Build history of the part. All positions in model axes, mm. A direction names the side the tool comes from. Give positions to 0.01 mm unless a question says otherwise; leave off trailing zeros. Order: outer loops, then holes, each group sorted by start corner. A loop starts at its lowest first (then second) coordinate and runs counter-clockwise, first axis right, second up. Notation, with made-up numbers: (3.5, 18) - (27.5, 18) arc R22 ccw to (27.5, 26) - close; hole circle Ø5 at (-14, 65). An arc over 180 degrees is marked (long way). Answer in a Markdown table with one row per item.
Autodesk Inventor part; units mm, degrees
ref_plane "YZ Plane" through (0, 0, 0) normal (1, 0, 0) x (0, 1, 0)
ref_plane "XZ Plane" through (0, 0, 0) normal (0, 1, 0) x (-1, 0, 0)
ref_plane "XY Plane" through (0, 0, 0) normal (0, 0, 1) x (1, 0, 0)
sketch "Sketch1" plane through (0, 0, 0) normal (0, 0, 1) x (1, 0, 0)
  line L0 (-51.8104, 0) -> (51.8104, 0) construction
  line L1 (0, -35.1144) -> (0, 36.3819) construction
  line L2 (0, 0) -> (26.1682, 26.1682) construction
  line L3 (0, 0) -> (37.0074, 0) construction
  line L4 (16.8, 24.9006) -> (16.8, 21.2406)
  line L5 (16.8, 21.2406) -> (19.0203, 19.0203)
  line L6 (16.8, 24.9006) -> (0, 24.9006)
  line L7 (24.9006, 16.8) -> (21.2406, 16.8)
  line L8 (21.2406, 16.8) -> (19.0203, 19.0203)
  line L9 (24.9006, 16.8) -> (24.9006, 0)
  line L10 (0, 0) -> (-37.0074, 0) construction
  line L11 (-16.8, 24.9006) -> (-16.8, 21.2406)
  line L12 (-16.8, 21.2406) -> (-19.0203, 19.0203)
  line L13 (-16.8, 24.9006) -> (0, 24.9006)
  line L14 (-24.9006, 16.8) -> (-24.9006, 0)
  line L15 (-24.9006, 16.8) -> (-21.2406, 16.8)
  line L16 (-21.2406, 16.8) -> (-19.0203, 19.0203)
  line L17 (16.8, -24.9006) -> (16.8, -21.2406)
  line L18 (16.8, -21.2406) -> (19.0203, -19.0203)
  line L19 (16.8, -24.9006) -> (0, -24.9006)
  line L20 (24.9006, -16.8) -> (24.9006, 0)
  line L21 (24.9006, -16.8) -> (21.2406, -16.8)
  line L22 (21.2406, -16.8) -> (19.0203, -19.0203)
  line L23 (-16.8, -24.9006) -> (-16.8, -21.2406)
  line L24 (-16.8, -21.2406) -> (-19.0203, -19.0203)
  line L25 (-16.8, -24.9006) -> (0, -24.9006)
  line L26 (-24.9006, -16.8) -> (-24.9006, 0)
  line L27 (-24.9006, -16.8) -> (-21.2406, -16.8)
  line L28 (-21.2406, -16.8) -> (-19.0203, -19.0203)
  line L29 (-16.8, -16.8) -> (16.8, 16.8) construction
  line L30 (17.4242, -17.4242) -> (-16.0391, 16.0391) construction
  line L31 (-16.8, -15) -> (16.8, -15)
  line L32 (16.8, -15) -> (16.8, 15)
  line L33 (16.8, 15) -> (-16.8, 15)
  line L34 (-16.8, 15) -> (-16.8, -15)
  line L35 (-16.8, -15) -> (16.8, 15) construction
  line L36 (16.8, -15) -> (-16.8, 15) construction
  dimension "d0" = 45
  dimension "d1" = 3.14
  dimension "d2" = 3.66
  dimension "d4" = 16.8
  dimension "d16" = 33.6
  dimension "d17" = 30
extrude "Extrusion1" add sketch "Sketch1" along normal blind 8
sketch "Sketch2" plane through (-16.8, 24.9006, 0) normal (0, 1, 0) x (1, 0, 0)
  line L0 (-8.1006, 0) -> (-4.4406, 0) construction
  line L1 (-8.1006, 0) -> (-8.1006, -8) construction
  line L2 (-4.4406, -8) -> (-8.1006, -8) construction
  line L3 (-4.4406, 0) -> (-4.4406, -8) construction
  line L4 (-4.4406, 0) -> (0, 0) construction
  line L5 (-4.4406, 0) -> (-4.4406, -8) construction
  line L6 (0, -8) -> (-4.4406, -8) construction
  line L7 (0, 0) -> (0, -8) construction
  line L8 (0, 0) -> (33.6, 0) construction
  line L9 (0, 0) -> (0, -8) construction
  line L10 (33.6, -8) -> (0, -8) construction
  line L11 (33.6, 0) -> (33.6, -8) construction
  line L12 (33.6, 0) -> (38.0406, 0) construction
  line L13 (33.6, 0) -> (33.6, -8) construction
  line L14 (38.0406, -8) -> (33.6, -8) construction
  line L15 (38.0406, 0) -> (38.0406, -8) construction
  line L16 (38.0406, 0) -> (41.7006, 0) construction
  line L17 (38.0406, 0) -> (38.0406, -8) construction
  line L18 (41.7006, -8) -> (38.0406, -8) construction
  line L19 (41.7006, 0) -> (41.7006, -8) construction
  line L20 (-0.9933, -0.6346) -> (2.8461, 5.7642) construction
  ellipse E0 centre (4.1754, 7.1215) end of major axis (2.3333, 6.6563) minor radius 1.8997 (5.4585, 5.7204) -> (2.8461, 5.7642) ccw construction
  line L21 (5.4585, 5.7204) -> (9.3415, -1.2728) construction
  line L22 (9.3415, -1.2728) -> (8.4179, -1.2574) construction
  line L23 (8.4179, -1.2574) -> (4.8304, 5.2036) construction
  ellipse E1 centre (5.2675, 5.4463) end of major axis (4.7828, 5.3239) minor radius 0.4999 (4.9945, 5.8651) -> (4.8304, 5.2036) ccw construction
  ellipse E2 centre (4.1754, 7.1215) end of major axis (2.7211, 6.7542) minor radius 1.4998 (4.9945, 5.8651) -> (3.3146, 5.8932) ccw construction
  ellipse E3 centre (3.0277, 5.4838) end of major axis (3.5125, 5.6062) minor radius 0.4999 (3.4564, 5.2266) -> (3.3146, 5.8932) ccw construction
  line L24 (3.4564, 5.2266) -> (-0.3461, -1.1107) construction
  ellipse E4 centre (-1.5262, -2.0366) end of major axis (-0.0719, -1.6693) minor radius 1.4998 (-0.9933, -0.6346) -> (-0.3461, -1.1107) ccw construction
  circle A0 centre (-2.1474, -2.1474) radius 1.7
  line L25 (-4.4406, 0) -> (0, 0) construction
  line L26 (0, 0) -> (-3.5302, -3.5302) construction
  line L27 (0, 0) -> (4.9925, 0) construction
  line L28 (0, 0) -> (2, 0)
  line L29 (0, 0) -> (-1.7777, 0)
  line L30 (-1.7777, 0) -> (-2.227, -0.4493)
  line L31 (0, 0) -> (0, -3.2892)
  line L32 (0, -3.2892) -> (-0.8879, -3.2892)
  point P0 (16.8, 0)
  dimension "d8" = 3.4
  dimension "d9" = 135
extrude "Extrusion2" cut sketch "Sketch2" against normal up to surface (39.9006 mm away)
sketch "Sketch3" plane through (0, 0, 0) normal (0, 0, -1) x (-1, 0, 0)
  line L0 (16.8, 15) -> (16.8, 24.9006) construction
  line L1 (16.8, 24.9006) -> (-16.8, 24.9006) construction
  line L2 (-16.8, 24.9006) -> (-16.8, 21.2406) construction
  line L3 (-16.8, 21.2406) -> (-21.2406, 16.8) construction
  line L4 (-21.2406, 16.8) -> (-24.9006, 16.8) construction
  line L5 (-24.9006, 16.8) -> (-24.9006, -16.8) construction
  line L6 (-24.9006, -16.8) -> (-21.2406, -16.8) construction
  line L7 (-21.2406, -16.8) -> (-16.8, -21.2406) construction
  line L8 (-16.8, -21.2406) -> (-16.8, -24.9006) construction
  line L9 (-16.8, -24.9006) -> (16.8, -24.9006) construction
  line L10 (16.8, -24.9006) -> (16.8, -21.2406) construction
  line L11 (16.8, -21.2406) -> (21.2406, -16.8) construction
  line L12 (21.2406, -16.8) -> (24.9006, -16.8) construction
  line L13 (24.9006, -16.8) -> (24.9006, 16.8) construction
  line L14 (24.9006, 16.8) -> (21.2406, 16.8) construction
  line L15 (21.2406, 16.8) -> (18.5777, 19.4629) construction
  line L16 (21.2406, 16.8) -> (24.9006, 16.8) construction
  line L17 (24.9006, 16.8) -> (21.2406, 16.8)
  line L18 (18.5777, 19.4629) -> (18.5777, -15)
  line L19 (16.8, 21.2406) -> (21.2406, 16.8)
  line L20 (21.2406, 16.8) -> (16.8, 21.2406)
  line L21 (16.8, 21.2406) -> (16.8, 16.8)
  line L22 (16.8, 16.8) -> (21.2406, 16.8)
  line L23 (18.5777, 19.4629) -> (18.5777, -15)
  line L24 (18.5777, -15) -> (-16.8, -15)
  line L25 (-16.8, -15) -> (-16.8, 15)
  line L26 (-16.8, 15) -> (16.8, 15)
  point P0 (0, 0)
  point P1 (18.5777, -16.8)
extrude "Extrusion3" cut sketch "Sketch3" against normal blind 3.9
mirror "Mirror1" about plane through (0, 0, 0) normal (1, 0, 0) of "Extrusion3", "Extrusion2"
sketch "Sketch4" plane through (-16.8, -15, 8) normal (0, 1, 0) x (1, 0, 0)
  line L0 (-1.7777, 8) -> (35.3777, 8) construction
  line L1 (-1.7777, 8) -> (-2.227, 7.5507) construction
  arc A0 (-2.227, 7.5507) -> (-0.8879, 4.7108) centre (-2.1474, 5.8526) ccw construction
  line L2 (-0.8879, 4.7108) -> (0, 4.7108) construction
  line L3 (0, 4.7108) -> (0, 0) construction
  line L4 (33.6, 0) -> (0, 0) construction
  line L5 (33.6, 4.7108) -> (33.6, 0) construction
  line L6 (34.4879, 4.7108) -> (33.6, 4.7108) construction
  arc A1 (34.4879, 4.7108) -> (35.827, 7.5507) centre (35.7474, 5.8526) ccw construction
  line L7 (35.3777, 8) -> (35.827, 7.5507) construction
  circle A2 centre (35.7474, 5.8526) radius 1.7
  circle A3 centre (-2.1474, 5.8526) radius 1.7
  point P0 (16.8, 8)
extrude "Extrusion4" cut sketch "Sketch4" against normal blind 10
sketch "Sketch5" plane through (-16.8, 24.9006, 0) normal (0, 1, 0) x (1, 0, 0)
  line L0 (0, 0) -> (33.6, 0) construction
  line L1 (0, 0) -> (0, -8) construction
  line L2 (33.6, -8) -> (0, -8) construction
  line L3 (33.6, 0) -> (33.6, -8) construction
  line L4 (16.8, 0) -> (16.8, -8) construction
  line L5 (33.6, 0) -> (33.6, -8) construction
  line L6 (0, 0) -> (0, -8) construction
  line L7 (33.6, -4) -> (0, -4) construction
  line L8 (2.5, -4) -> (31.1, -4) construction
  line L9 (2.5, -5.75) -> (31.1, -5.75)
  line L10 (31.1, -2.25) -> (2.5, -2.25)
  arc A0 (2.5, -2.25) -> (2.5, -5.75) centre (2.5, -4) ccw
  arc A1 (31.1, -5.75) -> (31.1, -2.25) centre (31.1, -4) ccw
  point P0 (16.8, -4)
  dimension "d20" = 3.5
  dimension "d21" = 2.5
extrude "Extrusion5" cut sketch "Sketch5" against normal through all
sketch "Sketch6" plane through (0, 0, 8) normal (0, 0, 1) x (1, 0, 0)
  line L0 (-16.8, -15) -> (-16.8, 15)
  line L1 (-16.8, 15) -> (16.8, 15)
  line L2 (16.8, 15) -> (16.8, -15)
  line L3 (16.8, -15) -> (-16.8, -15)
  line L4 (16.8, 21.2406) -> (16.8, 24.9006)
  line L5 (16.8, 24.9006) -> (-16.8, 24.9006)
  line L6 (-16.8, 24.9006) -> (-16.8, 21.2406)
  line L7 (-16.8, 21.2406) -> (-21.2406, 16.8)
  line L8 (-21.2406, 16.8) -> (-24.9006, 16.8)
  line L9 (-24.9006, 16.8) -> (-24.9006, -16.8)
  line L10 (-24.9006, -16.8) -> (-21.2406, -16.8)
  line L11 (-21.2406, -16.8) -> (-16.8, -21.2406)
  line L12 (-16.8, -21.2406) -> (-16.8, -24.9006)
  line L13 (-16.8, -24.9006) -> (16.8, -24.9006)
  line L14 (16.8, -24.9006) -> (16.8, -21.2406)
  line L15 (16.8, -21.2406) -> (21.2406, -16.8)
  line L16 (21.2406, -16.8) -> (24.9006, -16.8)
  line L17 (24.9006, -16.8) -> (24.9006, 16.8)
  line L18 (24.9006, 16.8) -> (21.2406, 16.8)
  line L19 (21.2406, 16.8) -> (16.8, 21.2406)
  point P0 (0, 0)
extrude "Extrusion6" cut sketch "Sketch6" against normal blind 2.1
properties part number "20_Rect_Aperture_Insert_half"
1. Two-plate mould, pull along Y, no slides. Class faces 1 (the face through (18, 18, 3.9)), 2 (the face through (-19.05, 18.99, 4.89)), 3 (the face through (16.8, 0, 5)), 4 (the face through (-16.8, 0, 5)): +Y half, -Y half, draft (parallel to the pull), parting line (faces both ways), or undercut.
Check result:
| item | result |
|---|---|
| face 1 | draft |
| face 2 | +Y half |
| face 3 | undercut |
| face 4 | undercut |
2. Cut at D-D on y = 18. Write the cut outline in (x, z).
Check result:
| item | result |
|---|---|
| outline | (-20.04, 3.9) - (-16.8, 3.9) - (-16.8, 0) - (16.8, 0) - (16.8, 3.9) - (20.04, 3.9) - (20.04, 5.9) - (-20.04, 5.9) - close; hole (-14.3, 2.25) - (14.3, 2.25) arc R1.75 ccw to (14.3, 5.75) - (-14.3, 5.75) arc R1.75 ccw to start |
3. Cut at B-B on z = 5.1. Write the cut outline in (x, y), and give its area (3 significant figures).
Check result:
| item | result |
|---|---|
| outline | (-24.9, -16.8) - (-21.24, -16.8) - (-16.8, -21.24) - (-16.8, -24.9) - (-15.66, -24.9) - (-15.66, -15) - (-16.8, -15) - (-16.8, 15) - (-15.66, 15) - (-15.66, 24.9) - (-16.8, 24.9) - (-16.8, 21.24) - (-21.24, 16.8) - (-24.9, 16.8) - close; (15.66, -24.9) - (16.8, -24.9) - (16.8, -21.24) - (21.24, -16.8) - (24.9, -16.8) - (24.9, 16.8) - (21.24, 16.8) - (16.8, 21.24) - (16.8, 24.9) - (15.66, 24.9) - (15.66, 15) - (16.8, 15) - (16.8, -15) - (15.66, -15) - close |
| area | 629 mm² |
4. Cut at C-C on y = -16. Write the cut outline in (x, z).
Check result:
| item | result |
|---|---|
| outline | (-24.9, 0) - (24.9, 0) - (24.9, 5.9) - (-24.9, 5.9) - close; hole circle Ø3.4 at (-18.95, 2.15); hole (-14.3, 2.25) - (14.3, 2.25) arc R1.75 ccw to (14.3, 5.75) - (-14.3, 5.75) arc R1.75 ccw to start; hole circle Ø3.4 at (18.95, 2.15) |
5. Probe line 1 (Z direction, x = 8.5, y = 21); line 2 (X direction, y = -2, z = 4.5); line 3 (X direction, y = -15.5, z = 1). List the from-to ranges inside material, lowest first.
Check result:
| item | result |
|---|---|
| line 1 | z = 0 to 2.25, 5.75 to 5.9 |
| line 2 | x = -24.9 to -16.8, 16.8 to 24.9 |
| line 3 | x = -24.9 to -20.2, -17.69 to 17.69, 20.2 to 24.9 |
6. Cut at A-A on y = 6. Write the cut outline in (x, z), and give its area (3 significant figures).
Check result:
| item | result |
|---|---|
| outline | (-24.9, 0) - (-18.58, 0) - (-19.03, 0.45) arc R1.7 cw (long way) to (-17.69, 3.29) - (-16.8, 3.29) - (-16.8, 5.9) - (-24.9, 5.9) - close; (16.8, 3.29) - (17.69, 3.29) arc R1.7 cw (long way) to (19.03, 0.45) - (18.58, 0) - (24.9, 0) - (24.9, 5.9) - (16.8, 5.9) - close |
| area | 71.5 mm² |
7. Which spindle directions (+Z, -Z, +X, -X, +Y, -Y) get a long thin tool onto all of the face, cutting with end or side? Do faces 5 (the face through (23, -16.8, 3)), 6 (the face through (-16.8, 21, 2)), 7 (the face through (-23, 16.8, 3)). Say none if no direction does.
Check result:
| item | result |
|---|---|
| face 5 | +Z, -Z, +X, -Y |
| face 6 | -Z, +Y |
| face 7 | -Z, -X, +Y |
8. Drop flat-ended pins along their axis: P1, Ø1, axis at x = 17, y = 3, coming from the -Z side; P2, Ø11, axis at x = 2.5, y = 21, coming from the -Z side; P3, Ø1.8, axis at x = -19, z = 2.5, coming from the +Y side; P4, Ø1.8, axis at y = -22.5, z = 4, coming from the +X side. Give the stop position or say it passes through.
Check result:
| item | result |
|---|---|
| P1 | stops at z = 3.29 |
| P2 | stops at z = 0 |
| P3 | passes through |
| P4 | stops at x = 16.8 |
